Could you check a few things on this model? Use its own coordinates, in mm. Face numbers are marked on the shaded views. A direction names the side the tool comes from. Give positions to 0.01 mm unless a question says otherwise; leave off trailing zeros. Order: outer loops, then holes, each group sorted by start corner. A loop starts at its lowest first (then second) coordinate and runs counter-clockwise, first axis right, second up. Notation, with made-up numbers: M 72.5,-10 L 131.5,-10 A11 cw 131.5,4 Z; hole C -4.75,36 d8. An arc over 180 degrees is marked long. Return JSON: item names as keys, results as strings. Group by question number.
```python
from build123d import *

# Parameters (mm, degrees)
SKETCH1_W           = 9.5
SKETCH1_H           = 4.5
BOSS_EXTRUDE1_DEPTH = 1.2
BOSS_EXTRUDE2_DEPTH = 4.5
SKETCH4_W           = 3.5
SKETCH4_H           = 0.9
CUT_EXTRUDE2_DEPTH  = 4.5
FILLET2_R           = 0.4
FILLET3_R           = 1


with BuildPart() as part:
    # Sketch1 → Boss-Extrude1 (new body)
    with BuildSketch(Plane(origin=(0, 3.3, 0), x_dir=(1, 0, 0), z_dir=(0, 1, 0))):
        with Locations((0, 0.35)):
            Rectangle(SKETCH1_W, SKETCH1_H)
    extrude(amount=-BOSS_EXTRUDE1_DEPTH)

    # Sketch2 → Boss-Extrude2 (add)
    with BuildSketch(Plane.XZ.offset(-2.1)):
        Polygon((3.425, -0.13), (2.65, -0.9), (-2.65, -0.9), (-3.425, -0.13), (-3.425, 0.9), (3.425, 0.9), align=None)
    extrude(amount=BOSS_EXTRUDE2_DEPTH)

    # Sketch4 → Cut-Extrude2 (cut)
    with BuildSketch(Plane.XZ.offset(2.4)):
        with Locations((0, 0.45)):
            Rectangle(SKETCH4_W, SKETCH4_H)
    extrude(amount=-CUT_EXTRUDE2_DEPTH, mode=Mode.SUBTRACT)

    # Fillet2
    fillet2_edges = [part.edges().sort_by_distance(p)[0] for p in [
        (3.425, -0.15, -0.13),
        (3.425, -0.15, 0.9),
        (-3.425, -0.15, 0.9),
        (-3.425, -0.15, -0.13),
        (-2.65, -0.15, -0.9),
        (2.65, -0.15, -0.9),
    ]]
    fillet(fillet2_edges, radius=FILLET2_R)

    # Fillet3
    fillet3_edges = [part.edges().sort_by_distance(p)[0] for p in [
        (-4.75, 2.7, 1.9),
        (-4.75, 2.7, -2.6),
        (4.75, 2.7, -2.6),
        (4.75, 2.7, 1.9),
    ]]
    fillet(fillet3_edges, radius=FILLET3_R)


solid = part.part
```
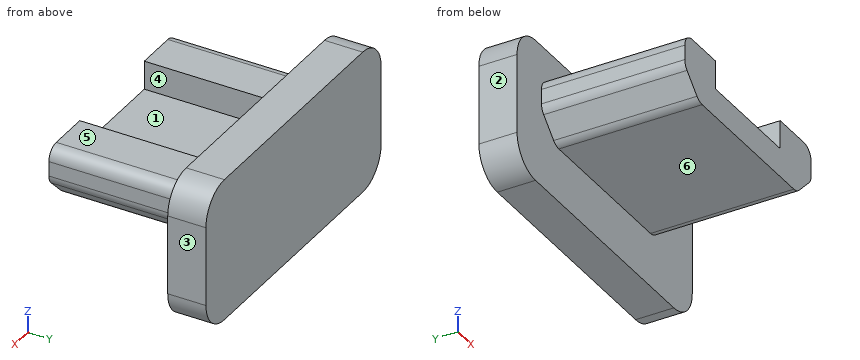
1. I need wall thicknesses on L1, parallel to X at y = -1.7, z = 0.2 (3 decimals); L2, parallel to Y at x = 3.75, z = -0.55; L3, parallel to Z at x = -0.25, y = 0.4. Which ranges of each line are inside material? Lowest first, please. Write a range as from..to.
2. Which directions (+Z, -Z, +X, -X, +Y, -Y) give clear straight access to the entire face, cutting with the end or side of a thin tool? Please do the marked faces 4, 5 and 6.
3. For pin 1 (1.5 mm diameter, centred on x = 2.5, y = -1.5, fed in from -Z); pin 2 (1.4 mm diameter, centred on x = 2, y = -1, fed in from +Z); pin 3 (1 mm diameter, centred on y = 0, z = 0.5, fed in from +X) (3 decimals), each with a flat end and sliding along its axis, tell me the tip position at first contact or that it passes through.
4. If we mould it in two halves opening along X, with no side actions, what happens to the marked faces 1, 2 and 3? For each: pulls with the +X half, pulls with the -X half, needs draft (parallel to the pull), parting line crosses it, or undercut.
5. Imagine slicing it at B-B, the plane x = -1.5. Please give me the cut outline in (y, z), plus the area to 3 significant figures.
6. Imagine slicing it at D-D, the plane z = -1. Please give me the cut outline in (x, y).
7. Imagine slicing it at A-A, the plane z = 0.4. Please give me the cut outline in (x, y) (3 decimals).
8. Imagine slicing it at C-C, the plane y = -0.9. Please give me the cut outline in (x, z) (3 decimals), plus the area to 3 significant figures.
Values:
{
 "1": {"L1": "x = -3.425..-1.75, 1.75..3.425", "L2": "y = 2.1..3.3", "L3": "z = -0.9..0"},
 "2": {"face 4": "+Z, -Y", "face 5": "+Z, +X, -X, -Y", "face 6": "-Z, +X, -X, -Y"},
 "3": {"pin 1": "stops at z = -0.9", "pin 2": "stops at z = 0.9", "pin 3": "stops at x = 3.425"},
 "4": {"face 1": "undercut", "face 2": "pulls with the -X half", "face 3": "pulls with the +X half"},
 "5": {"outline": "M -2.4,-0.9 L 2.1,-0.9 L 2.1,-2.6 L 3.3,-2.6 L 3.3,1.9 L 2.1,1.9 L 2.1,0 L -2.4,0 Z", "area": "9.45 mm²"},
 "6": {"outline": "M -4.75,2.1 L 4.75,2.1 L 4.75,3.3 L -4.75,3.3 Z"},
 "7": {"outline": "M -4.75,2.1 L -3.425,2.1 L -3.425,-2.4 L -1.75,-2.4 L -1.75,2.1 L 1.75,2.1 L 1.75,-2.4 L 3.425,-2.4 L 3.425,2.1 L 4.75,2.1 L 4.75,3.3 L -4.75,3.3 Z"},
 "8": {"outline": "M -3.425,0.036 A0.4 ccw -3.307,-0.247 L -2.767,-0.784 A0.4 ccw -2.485,-0.9 L 2.485,-0.9 A0.4 ccw 2.767,-0.784 L 3.307,-0.247 A0.4 ccw 3.425,0.036 L 3.425,0.5 A0.4 ccw 3.025,0.9 L 1.75,0.9 L 1.75,0 L -1.75,0 L -1.75,0.9 L -3.025,0.9 A0.4 ccw -3.425,0.5 Z", "area": "8.50 mm²"}
}
